Part print with two shaded views. Sizes in mm from the minimum x, y, z corner. Round coordinates to 2 decimals unless told otherwise and drop trailing zeros. Write each loop counter-clockwise with the first axis right and the second up, starting at its lowest first coordinate (ties: lowest second). Pieces come first, ordered by that corner, then holes. Notation, with made-up numbers: (55.25, -30.75) -> (97.25, -30.75) arc R13 ccw to (97.25, -22.75) -> close; hole circle Ø8 at (1, 18.25). An arc over 180 degrees is marked (long way). Return JSON: item names as keys, results as strings.
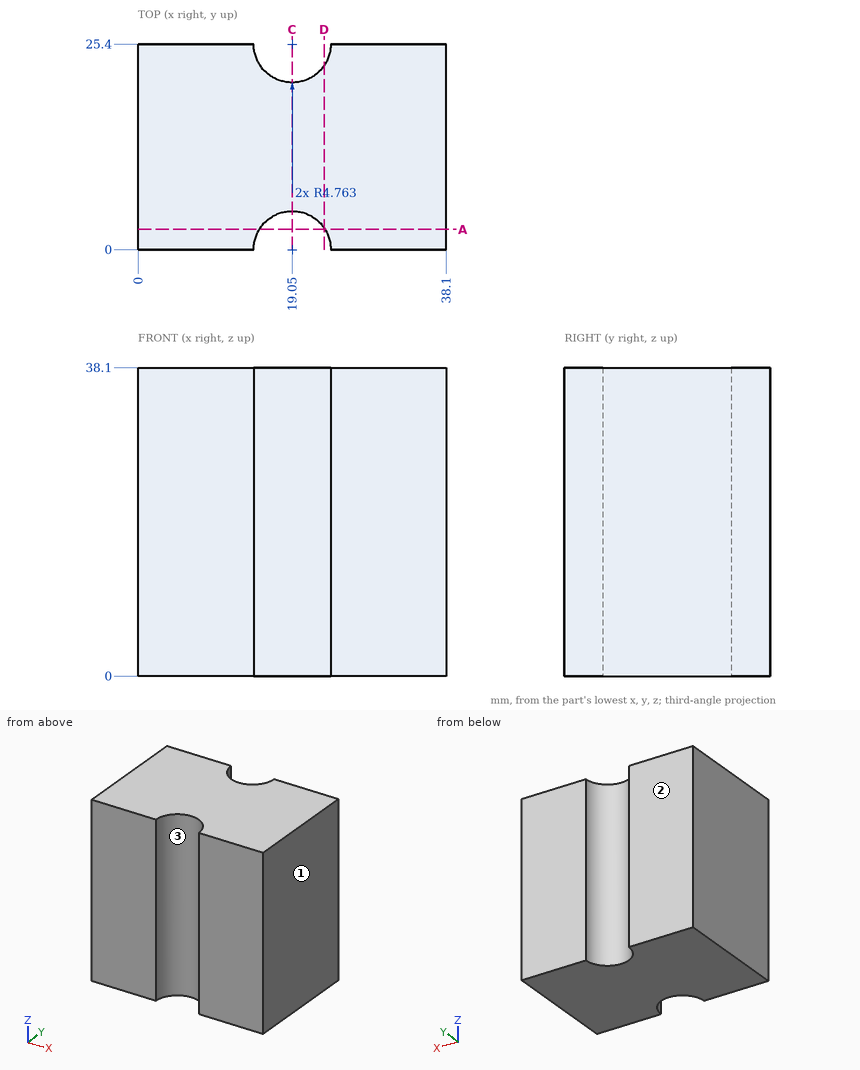
Q1. Saw through at C-C on x = 19.05. List the corners of the cut face in (y, z).
Verdict:
{"outline": "(4.76, 0) -> (20.64, 0) -> (20.64, 38.1) -> (4.76, 38.1) -> close"}
Q2. Two-plate mould, pull along X, no slides. Class the marked faces 1, 2 and 3: +X half, -X half, draft (parallel to the pull), parting line (faces both ways), or undercut.
Verdict:
{"face 1": "+X half", "face 2": "draft", "face 3": "undercut"}
Q3. Wall check: L1, parallel to X at y = 22.5, z = 10; L2, parallel to Y at x = 21, z = 30 (1 decimal); L3, parallel to X at y = 24, z = 9. Give the ranges that are in metal, low to high.
Verdict:
{"L1": "x = 0 to 15.27, 22.83 to 38.1", "L2": "y = 4.3 to 21.1", "L3": "x = 0 to 14.5, 23.6 to 38.1"}
Q4. Saw through at D-D on x = 23. List the corners of the cut face in (y, z).
Verdict:
{"outline": "(2.66, 0) -> (22.74, 0) -> (22.74, 38.1) -> (2.66, 38.1) -> close"}
Q5. Saw through at A-A on y = 2.5. List the corners of the cut face in (x, z).
Verdict:
{"outline": "(0, 0) -> (15, 0) -> (15, 38.1) -> (0, 38.1) -> close; (23.1, 0) -> (38.1, 0) -> (38.1, 38.1) -> (23.1, 38.1) -> close"}
